Here's how the part is built. I have some questions about the finished solid (model axes, mm). Face numbers are marked on the shaded views. A direction names the side the tool comes from. Round coordinates to 2 decimals unless told otherwise and drop trailing zeros. Write each loop counter-clockwise with the first axis right and the second up, starting at its lowest first coordinate (ties: lowest second). Pieces come first, ordered by that corner, then holes. Notation, with made-up numbers: (7.5, 70) - (14.5, 70) arc R10 cw to (14.5, 83) - close; hole circle Ø7 at (72.5, 53.25). An arc over 180 degrees is marked (long way). Use one line per item in the form item = value. Start each with the question number.
1. I want a section at B-B, the plane x = 0. List the corners of the cut face in (y, z) for me.
2. Which directions (+Z, -Z, +X, -X, +Y, -Y) give clear straight access to the entire face, cutting with the end or side of a thin tool? Please do the marked faces 1, 2 and 3.
3. If I drill on line 1 along Y through (x, z) = (-9.5, 9.5); line 2 along Y through (x, z) = (-11.5, -15); line 3 along X through (y, z) = (15.5, -23), over which ranges is the centre line in solid material (lowest first)?
4. I want a section at D-D, the plane y = -21. List the corners of the cut face in (x, z) for me, plus the area to 3 significant figures.
5. I want a section at A-A, the plane z = 0. List the corners of the cut face in (x, y) for me.
6. Will these pins go through, and if not, where does the flat tip stop? pin 1 (10 mm diameter, centred on x = 13, y = -3, fed in from -Z); pin 2 (4 mm diameter, centred on x = 15.5, z = 0, fed in from -Y); pin 3 (6 mm diameter, centred on x = 21.5, z = 5.5, fed in from -Y).
7. I want a section at C-C, the plane y = -3. List the corners of the cut face in (x, z) for me.
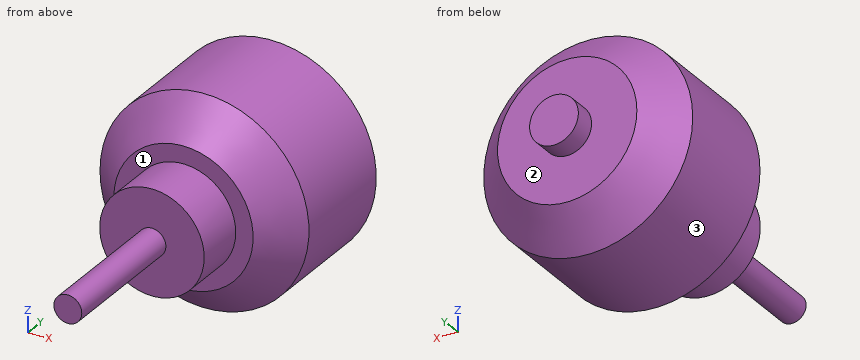
Autodesk Inventor part; units mm, degrees
ref_plane "YZ Plane" through (0, 0, 0) normal (1, 0, 0) x (0, 1, 0)
ref_plane "XZ Plane" through (0, 0, 0) normal (0, 1, 0) x (-1, 0, 0)
ref_plane "XY Plane" through (0, 0, 0) normal (0, 0, 1) x (1, 0, 0)
sketch "Sketch1" plane through (0, 0, 0) normal (0, 1, 0) x (-1, 0, 0)
  circle A0 centre (0, 0) radius 30
  dimension "d0" = 60
extrude "Extrusion1" add sketch "Sketch1" along normal blind 52
sketch "Sketch2" plane through (0, 52, 0) normal (0, 1, 0) x (1, 0, 0)
  circle A0 centre (0, 0) radius 7
  dimension "d3" = 14
extrude "Extrusion2" add sketch "Sketch2" along normal blind 6.3
sketch "Sketch3" plane through (0, 0, 0) normal (0, -1, 0) x (1, 0, 0)
  circle A0 centre (0, 0) radius 15
  dimension "d6" = 30
extrude "Extrusion3" add sketch "Sketch3" along normal blind 15
sketch "Sketch4" plane through (0, -15, 0) normal (0, -1, 0) x (1, 0, 0)
  circle A0 centre (0, 0) radius 4
  dimension "d9" = 8
extrude "Extrusion4" add sketch "Sketch4" along normal blind 40
chamfer "Chamfer1" distance 10 angle 45 1 edges at (30, 0, 0)
chamfer "Chamfer2" distance 10 angle 45 1 edges at (30, 52, 0)
properties part number "KV200_T_Motor"
Model answer:
q1.outline = (-55, -4) - (-15, -4) - (-15, -15) - (0, -15) - (0, -20) - (10, -30) - (42, -30) - (52, -20) - (52, -7) - (58.3, -7) - (58.3, 7) - (52, 7) - (52, 20) - (42, 30) - (10, 30) - (0, 20) - (0, 15) - (-15, 15) - (-15, 4) - (-55, 4) - close
q2.face_1 = -Y
q2.face_2 = +Y
q2.face_3 = +Y, -Y
q3.line_1 = -15 to 52
q3.line_2 = 0 to 52
q3.line_3 = -19.26 to 19.26
q4.outline = circle Ø8 at (0, 0)
q4.area = 50.3 mm2
q5.outline = (-30, 10) - (-20, 0) - (-15, 0) - (-15, -15) - (-4, -15) - (-4, -55) - (4, -55) - (4, -15) - (15, -15) - (15, 0) - (20, 0) - (30, 10) - (30, 42) - (20, 52) - (7, 52) - (7, 58.3) - (-7, 58.3) - (-7, 52) - (-20, 52) - (-30, 42) - close
q6.pin_1 = -18.58
q6.pin_2 = -15
q6.pin_3 = 0
q7.outline = circle Ø30 at (0, 0)
